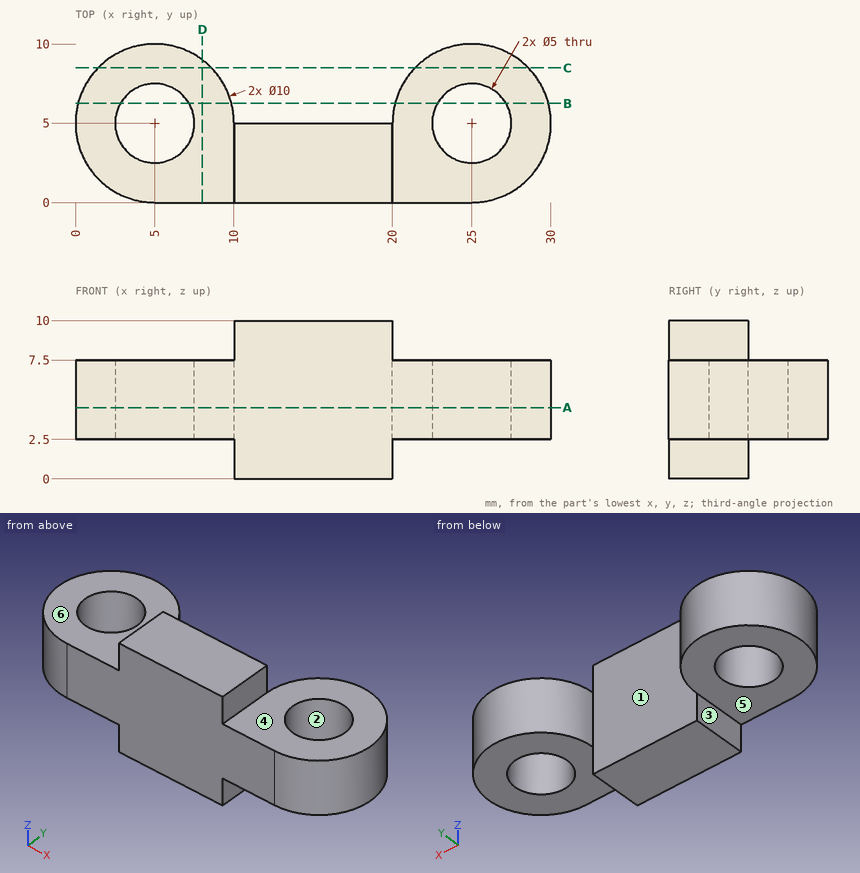
Could you check a few things on this drawing? It's one solid part, dimensions in mm from its lowest x, y, z. A direction names the side the tool comes from. Give positions to 0.01 mm unless a question says otherwise; leave off trailing zeros. Order: outer loops, then holes, each group sorted by start corner. A loop starts at its lowest first (then second) coordinate and runs counter-clockwise, first axis right, second up. Notation, with made-up numbers: (23, -16.75) - (73, -16.75) arc R17 ccw to (73, -1.75) - close; hole circle Ø8 at (68, 71). An arc over 180 degrees is marked (long way). Return JSON: item names as keys, results as strings. Group by question number.
Q1. Suppose I cut it at D-D, the plane x = 8. Please give me the cut outline in (y, z).
Q2. Suppose I cut it at C-C, the plane y = 8.5. Please give me the cut outline in (x, z).
Q3. Thinking about a two-plate mould opening in Y: for the marked faces 1, 2 and 3, which applies, pulls with the +Y half, pulls with the -Y half, needs draft (parallel to the pull), parting line crosses it, or undercut?
Q4. Suppose I cut it at A-A, the plane z = 4.5. Please give me the cut outline in (x, y).
Q5. Will these pins go through, and if not, where does the flat tip stop? pin 1 Ø1 at (x, y) = (4.5, 1) entering from +Z; pin 2 Ø2 at (y, z) = (2.5, 1) entering from +X; pin 3 Ø3 at (x, y) = (5, 3.5) entering from -Z.
Q6. Which directions (+Z, -Z, +X, -X, +Y, -Y) give clear straight access to the entire face, cutting with the end or side of a thin tool? Please do the marked faces 4, 5 and 6.
Q7. Suppose I cut it at B-B, the plane y = 6.25. Please give me the cut outline in (x, z), and give its area (3 significant figures).
Q8. Please list where these lines run through material, in increasing order: line 1 along X through (y, z) = (6.5, 6.5); line 2 along X through (y, z) = (1.25, 8.5); line 3 along Z through (x, y) = (5.5, 8.25). Write a range as [from, to].
Resolved:
{
 "1": {"outline": "(0, 2.5) - (9, 2.5) - (9, 7.5) - (0, 7.5) - close"},
 "2": {"outline": "(1.43, 2.5) - (8.57, 2.5) - (8.57, 7.5) - (1.43, 7.5) - close; (21.43, 2.5) - (28.57, 2.5) - (28.57, 7.5) - (21.43, 7.5) - close"},
 "3": {"face 1": "pulls with the +Y half", "face 2": "undercut", "face 3": "needs draft"},
 "4": {"outline": "(5, 0) - (25, 0) arc R5 ccw (long way) to (20, 5) - (10, 5) arc R5 ccw (long way) to start; hole circle Ø5 at (5, 5); hole circle Ø5 at (25, 5)"},
 "5": {"pin 1": "stops at z = 7.5", "pin 2": "stops at x = 20", "pin 3": "stops at z = 2.5"},
 "6": {"face 4": "+Z, +X, +Y, -Y", "face 5": "-Z, -X, +Y, -Y", "face 6": "+Z, -X, +Y, -Y"},
 "7": {"outline": "(0.16, 2.5) - (2.83, 2.5) - (2.83, 7.5) - (0.16, 7.5) - close; (7.17, 2.5) - (9.84, 2.5) - (9.84, 7.5) - (7.17, 7.5) - close; (20.16, 2.5) - (22.83, 2.5) - (22.83, 7.5) - (20.16, 7.5) - close; (27.17, 2.5) - (29.84, 2.5) - (29.84, 7.5) - (27.17, 7.5) - close", "area": "53.5 mm2"},
 "8": {"line 1": "x = [0.23, 3], [7, 9.77], [20.23, 23], [27, 29.77]", "line 2": "x = [10, 20]", "line 3": "z = [2.5, 7.5]"}
}
